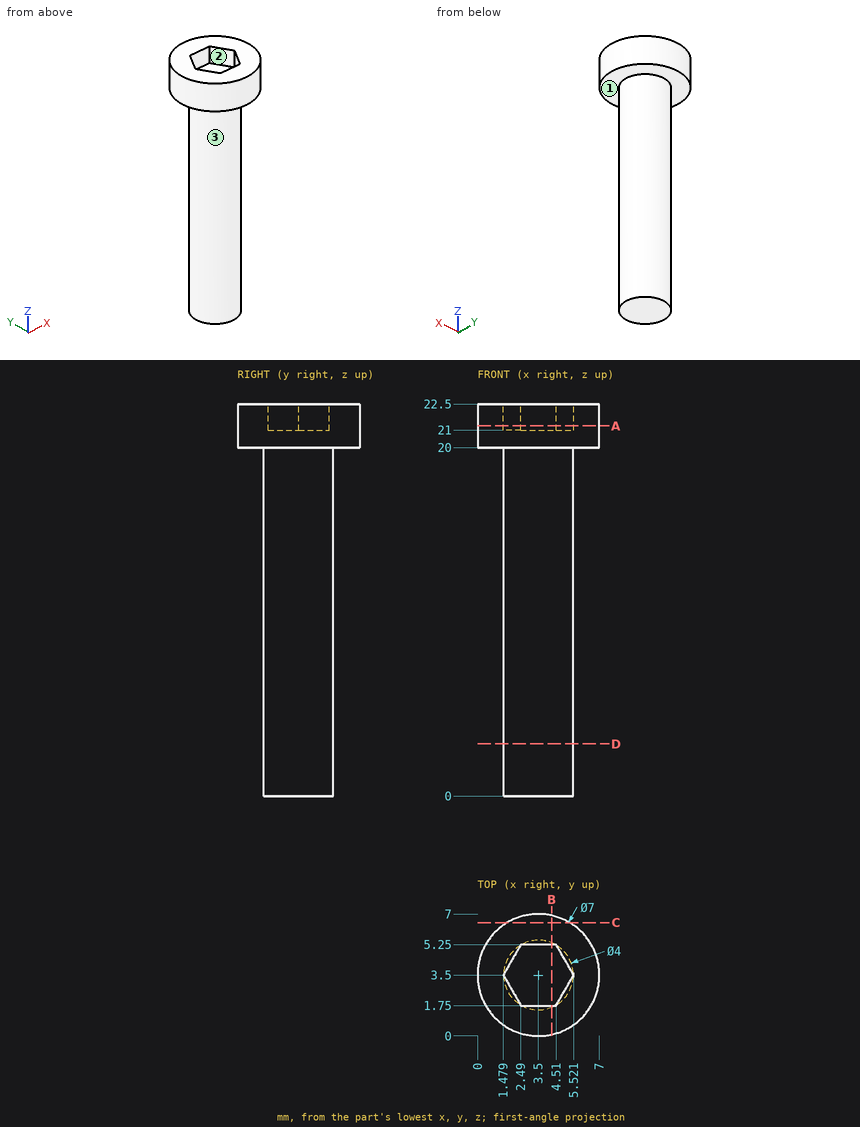
Print and shaded views of the part. All mm, measured from the part's lowest x, y and z. Give positions to 0.01 mm unless a question says otherwise; leave off trailing zeros. Loops run counter-clockwise (first coordinate to the right, second up) from the corner with the lowest first, then second, coordinate; pieces in that order, holes last. Notation, with made-up numbers: (-37.5, 55.25) - (-24.5, 55.25) arc R16 cw to (-24.5, 69.25) - close; hole circle Ø2 at (26, 17.25). An arc over 180 degrees is marked (long way). Use a Markdown table: item, result.
(1) Pull direction X, two halves, no side cores. Call the marked faces 1, 2 and 3: +X half, -X half, draft (parallel to the pull), parting line (faces both ways), or undercut.
Taken from the geometry:
| item | result |
|---|---|
| face 1 | draft |
| face 2 | undercut |
| face 3 | parting line |
(2) Drop flat-ended pins along their axis: pin 1 Ø4 at (y, z) = (2.5, 13.5) entering from -X; pin 2 Ø1 at (y, z) = (1.5, 15.5) entering from -X; pin 3 Ø1.5 at (x, z) = (2.5, 2.5) entering from +Y. Give the stop position or say it passes through.
Taken from the geometry:
| item | result |
|---|---|
| pin 1 | x = 1.5 |
| pin 2 | x = 2.18 |
| pin 3 | y = 5.48 |
(3) Band-saw the part on D-D (z = 3). Give the cut face in (x, y), and give its area (3 significant figures).
Taken from the geometry:
| item | result |
|---|---|
| outline | circle Ø4 at (3.5, 3.5) |
| area | 12.6 mm2 |
(4) Wall check: line 1 along X through (y, z) = (3.5, 7.75); line 2 along Z through (x, y) = (3, 3); line 3 along Z through (x, y) = (4.75, 5.75). Give the ranges that are in metal, low to high.
Taken from the geometry:
| item | result |
|---|---|
| line 1 | 1.5 to 5.5 |
| line 2 | 0 to 21 |
| line 3 | 20 to 22.5 |
(5) Band-saw the part on C-C (y = 6.5). Give the cut face in (x, z).
Taken from the geometry:
| item | result |
|---|---|
| outline | (1.7, 20) - (5.3, 20) - (5.3, 22.5) - (1.7, 22.5) - close |
(6) Band-saw the part on A-A (z = 21.25). Give the cut face in (x, y), and give its area (3 significant figures).
Taken from the geometry:
| item | result |
|---|---|
| outline | circle Ø7 at (3.5, 3.5); hole (1.48, 3.5) - (2.49, 1.75) - (4.51, 1.75) - (5.52, 3.5) - (4.51, 5.25) - (2.49, 5.25) - close |
| area | 27.9 mm2 |
(7) Band-saw the part on B-B (x = 4.25). Give the cut face in (y, z).
Taken from the geometry:
| item | result |
|---|---|
| outline | (0.08, 20) - (1.65, 20) - (1.65, 0) - (5.35, 0) - (5.35, 20) - (6.92, 20) - (6.92, 22.5) - (5.25, 22.5) - (5.25, 21) - (1.75, 21) - (1.75, 22.5) - (0.08, 22.5) - close |
